Can you work these out from the drawing? Everything is in mm from the part's minimum corner. A direction names the side the tool comes from. Coordinates: 2 decimals unless noted, no trailing zeros. Loops run counter-clockwise (first coordinate to the right, second up) from the corner with the lowest first, then second, coordinate; pieces in that order, holes last. Notation, with made-up numbers: M 87,11.5 L 137,11.5 A27 ccw 137,29.5 Z; hole C -19.75,19 d6. An arc over 180 degrees is marked long. Use CSV: the item, a comma, the result in double quotes. Start each with the question number.
Q1. Please list where these lines run through material, in increasing order: probe 1 along Z at (x, y) = (4.5, 10.5) (3 decimals); probe 2 along Z at (x, y) = (4, 9.5) (3 decimals); probe 3 along Y at (x, z) = (3.5, 17.75) (3 decimals). Write a range as [from, to].
Q2. If we section it at B-B (z = 20.25): Please give me the cut outline in (x, y) (3 decimals), and give its area (3 significant figures).
Q3. Which directions (+Z, -Z, +X, -X, +Y, -Y) give clear straight access to the entire face, cutting with the end or side of a thin tool? Please do the marked faces 1 and 2.
Q4. If we section it at D-D (z = 15): Please give me the cut outline in (x, y) (3 decimals), and give its area (3 significant figures).
Q5. If we section it at C-C (x = 4): Please give me the cut outline in (y, z) (3 decimals), and give its area (3 significant figures).
Q6. If we section it at A-A (y = 11.43): Please give me the cut outline in (x, z) (3 decimals).
Q7. For pin 1 Ø1 at (x, z) = (5.5, 8.5) entering from +Y; pin 2 Ø2 at (x, y) = (2, 8.5) entering from -Z; pin 3 Ø1.9 at (x, z) = (4.5, 18) entering from +Y, each with a flat end and sliding along its axis, tell me the tip position at first contact or that it passes through.
Q8. If we mould it in two halves opening along Z, with no side actions, what happens to the marked faces 3, 4 and 5? For each: +Z half, -Z half, draft (parallel to the pull), parting line (faces both ways), or undercut.
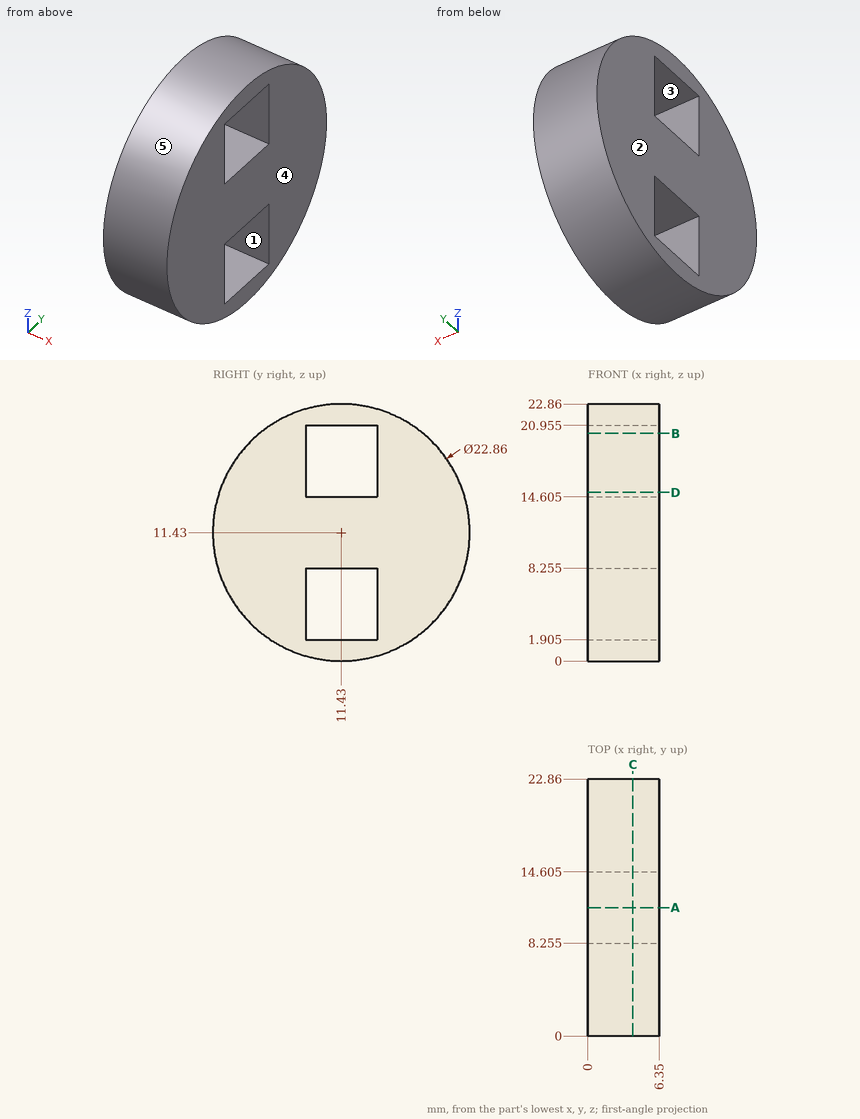
Results below:
1,probe 1,"[0.038, 1.905], [8.255, 14.605], [20.955, 22.822]"
1,probe 2,"[0.164, 1.905], [8.255, 14.605], [20.955, 22.696]"
1,probe 3,"[1.906, 8.255], [14.605, 20.954]"
2,outline,"M 0,4.16 L 6.35,4.16 L 6.35,8.255 L 0,8.255 Z; M 0,14.605 L 6.35,14.605 L 6.35,18.7 L 0,18.7 Z"
2,area,"52.0 mm^2"
3,face 1,"+X, -X"
3,face 2,"+Z, -Z, -X, +Y, -Y"
4,outline,"M 0,0.572 L 6.35,0.572 L 6.35,8.255 L 0,8.255 Z; M 0,14.605 L 6.35,14.605 L 6.35,22.288 L 0,22.288 Z"
4,area,"97.6 mm^2"
5,outline,"C 11.43,11.43 d22.86; hole M 8.255,1.905 L 14.605,1.905 L 14.605,8.255 L 8.255,8.255 Z; hole M 8.255,14.605 L 14.605,14.605 L 14.605,20.955 L 8.255,20.955 Z"
5,area,"330 mm^2"
6,outline,"M 0,0 L 6.35,0 L 6.35,1.905 L 0,1.905 Z; M 0,8.255 L 6.35,8.255 L 6.35,14.605 L 0,14.605 Z; M 0,20.955 L 6.35,20.955 L 6.35,22.86 L 0,22.86 Z"
7,pin 1,"y = 22.6"
7,pin 2,"z = 0.16"
7,pin 3,"y = 21.38"
8,face 3,"undercut"
8,face 4,"draft"
8,face 5,"parting line"
